Solid Edge part; units mm, degrees
sketch "Sketch1" plane through (0, 0, 0) normal (0, -1, 0) x (1, 0, 0)
  line L0 (0, 0) -> (0, 27)
  line L1 (2, 27) -> (0, 27)
  line L2 (2, 27) -> (2, 2)
  line L3 (2, 2) -> (37, 2)
  line L4 (37, 0) -> (37, 2)
  line L5 (0, 0) -> (37, 0)
extrude "Protrusion1" add sketch "Sketch1" along normal blind 24
sketch "Sketch2" plane through (0, -12, 13.5) normal (-1, 0, 0) x (0, -1, 0)
  line L0 (12, 1.5) -> (14.2005, 1.5)
  line L1 (14.2005, 1.5) -> (14.2005, 15.1309)
  line L2 (14.2005, 15.1309) -> (-13.515, 15.1309)
  line L3 (-13.515, 15.1309) -> (-13.515, 1.5)
  line L4 (-13.515, 1.5) -> (-12, 1.5)
  arc A0 (-12, 1.5) -> (12, 1.5) centre (0, 1.5) cw
extrude "ExtrudedCutout_1" cut sketch "Sketch2" against normal blind 10
sketch "Sketch3" plane through (0, -12, 13.5) normal (-1, 0, 0) x (0, -1, 0)
  circle A0 centre (0, 1.5) radius 1.5
  circle A1 centre (8.5, 1.5) radius 1.5
  circle A2 centre (-8.5, 1.5) radius 1.5
extrude "ExtrudedCutout_2" cut sketch "Sketch3" against normal blind 10
fillet "Round_1" radius 1 1 edges at (2, -12, 2)
sketch "Sketch4" plane through (18.5, 0, 7.5) normal (0, 1, 0) x (-1, 0, 0)
  line L0 (18.5, 7.5) -> (18.5, -7.5)
  line L1 (18.5, -7.5) -> (3.5, -7.5)
  line L2 (3.5, -7.5) -> (18.5, 7.5)
extrude "ExtrudedProtrusion_2" add sketch "Sketch4" along normal blind 2
sketch "Sketch5" plane through (18.5, -24, 7.5) normal (0, -1, 0) x (1, 0, 0)
  line L0 (-18.5, -7.5) -> (-18.5, 7.5)
  line L1 (-3.5, -7.5) -> (-18.5, 7.5)
  line L2 (-18.5, -7.5) -> (-3.5, -7.5)
extrude "ExtrudedProtrusion_3" add sketch "Sketch5" along normal blind 2
fillet "Round_2" radius 2 6 edges at (7.5, -26, 0) (7.5, 2, 0) (0, -26, 7.5) (0, 2, 7.5) (7.5, 2, 7.5) (7.5, -26, 7.5)
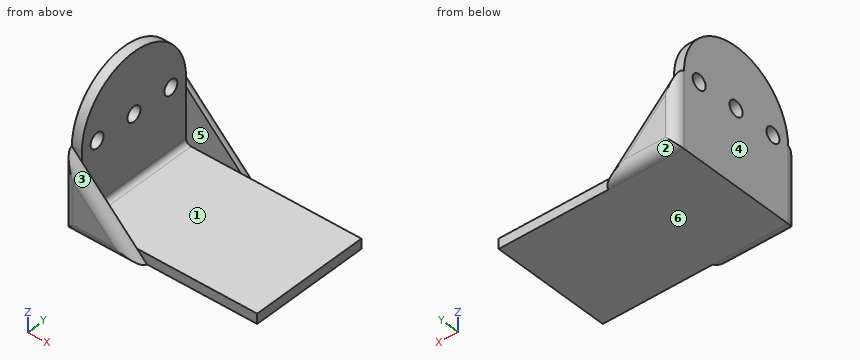
Input: part model. Units: mm. Frame: model coordinates. Face numbers are marked on the shaded views. A direction names the side the tool comes from. Give positions to 0.01 mm unless a question says otherwise; leave off trailing zeros. Write each loop counter-clockwise with the first axis right and the second up, starting at its lowest first coordinate (ties: lowest second). Pieces come first, ordered by that corner, then holes. Notation, with made-up numbers: (88, -29) - (146, -29) arc R21 ccw to (146, -1) - close; hole circle Ø10 at (71, 42.5). An arc over 180 degrees is marked (long way). Write item = value, one per line. Start each with the question number.
1. Section query D-D, the plane y = -8. Output: boundary loops of the cut face in (x, z).
2. First-contact query: pin 1 Ø0.6 at (x, z) = (29, 1.5) entering from -Y; pin 2 Ø3 at (x, y) = (4.5, -23) entering from -Z; pin 3 Ø12 at (x, y) = (15, -12) entering from +Z; pin 4 Ø1 at (x, z) = (24.5, 1) entering from +Y. Flat tips, straight axial feed; report the tip coordinate or a pass-through.
3. Section query B-B, the plane y = -19.75. Output: boundary loops of the cut face in (x, z).
4. Ray query, L1, parallel to Z at x = 0.7, y = -12; L2, parallel to Z at x = 9.5, y = -14.75. Return the intervals inside material, ascending.
5. Mould query, pull axis Y, two halves, no side actions, for the marked faces 1, 2, 3 and 4. Classes: released by +Y, released by -Y, zero draft, split by the parting line, or undercut.
6. Section query C-C, the plane x = 27. Output: boundary loops of the cut face in (y, z), then the cut area to 3 significant figures.
7. Access query for the marked faces 5 and 6. Directions: +Z, -Z, +X, -X, +Y, -Y. A direction counts if a zero-diameter tool reaches every point of the face in a straight line with its end or side. Return the directions, or none.
8. Section query A-A, the plane y = -12. Output: boundary loops of the cut face in (x, z).
Check sheet entries:
q1.outline = (0, 0) - (37, 0) - (37, 2) - (3, 2) arc R1 cw to (2, 3) - (2, 26.31) - (0, 26.31) - close
q2.pin_1 = -24
q2.pin_2 = 0
q2.pin_3 = 2
q2.pin_4 = 0
q3.outline = (0, 0) - (37, 0) - (37, 2) - (3, 2) arc R1 cw to (2, 3) - (2, 13.7) - (0, 13.7) - close; (0, 16.3) - (2, 16.3) - (2, 24.16) - (0, 24.16) - close
q4.L1 = 0 to 13.5, 16.5 to 27
q4.L2 = 0 to 2
q5.face_1 = undercut
q5.face_2 = released by +Y
q5.face_3 = released by -Y
q5.face_4 = zero draft
q6.outline = (-24, 0) - (0, 0) - (0, 2) - (-24, 2) - close
q6.area = 48.0 mm2
q7.face_5 = +Z, +X
q7.face_6 = -Z, +X, -X, +Y, -Y
q8.outline = (0, 0) - (37, 0) - (37, 2) - (3, 2) arc R1 cw to (2, 3) - (2, 13.5) - (0, 13.5) - close; (0, 16.5) - (2, 16.5) - (2, 27) - (0, 27) - close
